```python
from build123d import *

# Parameters (mm, degrees)
SKETCH1_R           = 4
BOSS_EXTRUDE1_DEPTH = 35
SKETCH3_W           = 44.253465858
SKETCH3_H           = 32.381458222
CUT_EXTRUDE1_DEPTH  = 27.5
SKETCH4_W           = 83.940233782
SKETCH4_H           = 63
CUT_EXTRUDE2_DEPTH  = 68.149087857
CHAMFER1_SIZE       = 10
SKETCH7_W           = 20
SKETCH7_H           = 18
CUT_EXTRUDE3_DEPTH  = 88.155034278
FILLET2_R           = 2
BOSS_EXTRUDE4_START = 1
BOSS_EXTRUDE4_DEPTH = 72
SKETCH11_R          = 1.5
BOSS_EXTRUDE5_DEPTH = 0.5


with BuildPart() as part:
    # Sketch1 → Boss-Extrude1 (new, symmetric)
    with BuildSketch(Plane.XY):
        with BuildLine():
            Line((-36, 14), (33, 14))
            Line((33, 14), (33, -14))
            Line((33, -14), (-36, -14))
            ThreePointArc((-36, -14), (-50, 0), (-36, 14))
        make_face()
        with Locations((-36, 0)):
            Circle(SKETCH1_R, mode=Mode.SUBTRACT)
    extrude(amount=BOSS_EXTRUDE1_DEPTH, both=True)

    # Sketch3 → Cut-Extrude1 (cut, symmetric)
    with BuildSketch(Plane.XY):
        with Locations((-36, 0)):
            Rectangle(SKETCH3_W, SKETCH3_H)
    extrude(amount=CUT_EXTRUDE1_DEPTH, both=True, mode=Mode.SUBTRACT)

    # Sketch4 → Cut-Extrude2 (cut, through all)
    with BuildSketch(Plane(origin=(0, 14, 0), x_dir=(1, 0, 0), z_dir=(0, 1, 0))):
        with Locations((-11.375607931, 0)):
            Rectangle(SKETCH4_W, SKETCH4_H)
    extrude(amount=-CUT_EXTRUDE2_DEPTH, mode=Mode.SUBTRACT)

    # Chamfer1
    chamfer1_edges = [part.edges().sort_by_distance(p)[0] for p in [
        (30.59450896, 0, 31.5),
        (30.59450896, 0, -31.5),
    ]]
    chamfer(chamfer1_edges, length=CHAMFER1_SIZE)

    # Sketch7 → Cut-Extrude3 (cut, through all)
    with BuildSketch(Plane.XY.offset(35)):
        with Locations((-17.198958596, 0)):
            Rectangle(SKETCH7_W, SKETCH7_H)
        with Locations((10.301041404, 0)):
            Rectangle(SKETCH7_W, SKETCH7_H)
    extrude(amount=-CUT_EXTRUDE3_DEPTH, mode=Mode.SUBTRACT)

    # Fillet2
    # the kernel refuses this fillet: 2 mm, written as the material it adds along each edge
    with BuildSketch(Plane(origin=(-27.198958596, -9, -31.5), x_dir=(0, 1, 0), z_dir=(0, 0, -1)), Plane(origin=(-7.198958596, 9, -31.5), x_dir=(0, -1, 0), z_dir=(0, 0, -1)), Plane(origin=(-7.198958596, 9, 35), x_dir=(0, -1, 0), z_dir=(0, 0, -1)), Plane(origin=(-7.198958596, -9, -31.5), x_dir=(-1, 0, 0), z_dir=(0, 0, -1)), Plane(origin=(0.301041404, -9, -31.5), x_dir=(0, 1, 0), z_dir=(0, 0, -1))) as fillet2_piece_1:
        with BuildLine():
            CenterArc((FILLET2_R, FILLET2_R), FILLET2_R, 180, 90)
            Line((0, FILLET2_R), (0, 0))
            Line((0, 0), (FILLET2_R, 0))
        make_face()
    extrude(amount=3.5)
    with BuildSketch(Plane(origin=(-27.198958596, -9, 35), x_dir=(1, 0, 0), z_dir=(0, 0, -1)), Plane(origin=(-27.198958596, 9, -31.5), x_dir=(0, -1, 0), z_dir=(0, 0, -1)), Plane(origin=(-27.198958596, 9, 35), x_dir=(0, -1, 0), z_dir=(0, 0, -1)), Plane(origin=(-7.198958596, -9, 35), x_dir=(0, 1, 0), z_dir=(0, 0, -1)), Plane(origin=(0.301041404, -9, 35), x_dir=(1, 0, 0), z_dir=(0, 0, -1)), Plane(origin=(0.301041404, 9, -31.5), x_dir=(0, -1, 0), z_dir=(0, 0, -1)), Plane(origin=(0.301041404, 9, 35), x_dir=(0, -1, 0), z_dir=(0, 0, -1))) as fillet2_piece_2:
        with BuildLine():
            CenterArc((FILLET2_R, -FILLET2_R), FILLET2_R, 90, 90)
            Line((0, -FILLET2_R), (0, 0))
            Line((0, 0), (FILLET2_R, 0))
        make_face()
    extrude(amount=3.5)
    # the kernel refuses this fillet: 2 mm, written as the material it takes off along each edge
    with BuildSketch(Plane(origin=(20.301041404, 9, -31.5), x_dir=(1, 0, 0), z_dir=(0, -1, 0)), Plane(origin=(20.301041404, -9, 31.5), x_dir=(1, 0, 0), z_dir=(0, 1, 0))) as fillet2_2_piece_1:
        with BuildLine():
            CenterArc((2, -1.042951109), FILLET2_R, 148.568719088, 31.431280912)
            Line((0, -1.042951109), (0, 0))
            Line((0, 0), (0.293467555, 0))
        make_face()
    extrude(amount=18, mode=Mode.SUBTRACT)

    # Sketch10 → Boss-Extrude4 (add)
    with BuildSketch(Plane.XY.offset(35).offset(BOSS_EXTRUDE4_START)):
        Polygon((33, 14), (34, 14), (34, 20.5), (35, 20.5), (35, 13), (33, 13), align=None)
        Polygon((33, -14), (33, -13), (35, -13), (35, -20.5), (34, -20.5), (34, -14), align=None)
    extrude(amount=-BOSS_EXTRUDE4_DEPTH)

    # Sketch11 → Boss-Extrude5 (add)
    with BuildSketch(Plane(origin=(33, 0, 0), x_dir=(0, 0, -1), z_dir=(1, 0, 0))):
        with Locations(Location((0, 0, 0), (0, 0, 270))):
            Circle(SKETCH11_R)
    extrude(amount=BOSS_EXTRUDE5_DEPTH)


solid = part.part
```
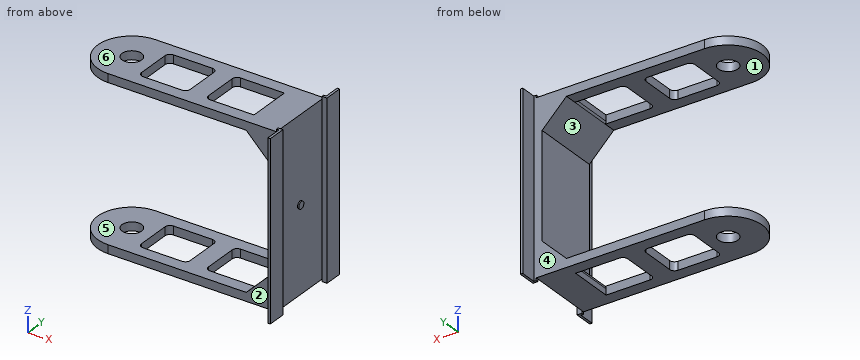
Geometry: final body of the model. Coordinates: model frame, mm. Face numbers are marked on the shaded views. A direction names the side the tool comes from. Coordinates: 2 decimals unless noted, no trailing zeros. Order: outer loops, then holes, each group sorted by start corner. A loop starts at its lowest first (then second) coordinate and runs counter-clockwise, first axis right, second up. Notation, with made-up numbers: (8, 44.5) - (28, 44.5) arc R18 ccw to (28, 74.5) - close; hole circle Ø9 at (49.25, 3.5). An arc over 180 degrees is marked (long way). Return JSON: item names as keys, results as strings. Group by question number.
1. Cut plane C-C (y = -5). Output: boundary loops of the cut face in (x, z).
2. Cut plane A-A (x = -16.5). Output: boundary loops of the cut face in (y, z), plus the area to 3 significant figures.
3. Set-up query: the marked faces 1 and 2. Return all of +Z, -Z, +X, -X, +Y, -Y with unobstructed straight access to the full face (end or side cutting, diameter ignored); none if empty.
4. Cut plane B-B (z = -19). Output: boundary loops of the cut face in (x, y).
5. Pull-direction query (Z, two-part tool) for the marked faces 3, 4, 5 and 6; classes: pulls with the +Z half, pulls with the -Z half, needs draft (parallel to the pull), parting line crosses it, or undercut.
6. Pin query (flat end, axial travel): pin 1 (1 mm diameter, centred on y = 2, z = -33.5, fed in from +X); pin 2 (3 mm diameter, centred on x = 16, y = 11.5, fed in from -Z); pin 3 (0.8 mm diameter, centred on y = -13.5, z = 35.5, fed in from -X); pin 4 (6.5 mm diameter, centred on x = -36, y = 0, fed in from -Z). Return the tip coordinate at first contact, or that it passes through.
7. Cut plane D-D (x = 27.5). Output: boundary loops of the cut face in (y, z), plus the area to 3 significant figures.
8. Material intervals for line 1 along X through (y, z) = (0, 32.75); line 2 along Y through (x, z) = (-36, 33.8); line 3 along Z through (x, y) = (-3, 1), sorted ascending. Write a range as [from, to].
Resolved:
{
 "1": {"outline": "(-49.08, -35) - (-27.2, -35) - (-27.2, -31.5) - (-49.08, -31.5) - close; (-49.08, 31.5) - (-27.2, 31.5) - (-27.2, 35) - (-49.08, 35) - close; (-7.2, -35) - (0.3, -35) - (0.3, -31.5) - (-7.2, -31.5) - close; (-7.2, 31.5) - (0.3, 31.5) - (0.3, 35) - (-7.2, 35) - close; (20.3, -35) - (33, -35) - (33, 35) - (20.3, 35) - (20.3, 32.54) arc R2 ccw to (20.59, 31.5) - (30.59, 21.5) - (30.59, -21.5) - (20.59, -31.5) arc R2 ccw to (20.3, -32.54) - close"},
 "2": {"outline": "(-14, -35) - (-9, -35) - (-9, -31.5) - (-14, -31.5) - close; (-14, 31.5) - (-9, 31.5) - (-9, 35) - (-14, 35) - close; (9, -35) - (14, -35) - (14, -31.5) - (9, -31.5) - close; (9, 31.5) - (14, 31.5) - (14, 35) - (9, 35) - close", "area": "70.0 mm²"},
 "3": {"face 1": "-X, +Y, -Y", "face 2": "+Z, -Z, -X, -Y"},
 "4": {"outline": "(30.59, -14) - (34, -14) - (34, -20.5) - (35, -20.5) - (35, -13) - (33, -13) - (33, 13) - (35, 13) - (35, 20.5) - (34, 20.5) - (34, 14) - (30.59, 14) - close"},
 "5": {"face 3": "undercut", "face 4": "needs draft", "face 5": "undercut", "face 6": "pulls with the +Z half"},
 "6": {"pin 1": "stops at x = 33", "pin 2": "stops at z = -35", "pin 3": "stops at x = 33", "pin 4": "passes through"},
 "7": {"outline": "(-14, -35) - (14, -35) - (14, -24.59) - (-14, -24.59) - close; (-14, 24.59) - (14, 24.59) - (14, 35) - (-14, 35) - close", "area": "583 mm²"},
 "8": {"line 1": "x = [-50, -40], [-32, -27.2], [-7.2, 0.3], [20.3, 33]", "line 2": "y = [-14, -4], [4, 14]", "line 3": "z = [-35, -31.5], [31.5, 35]"}
}
